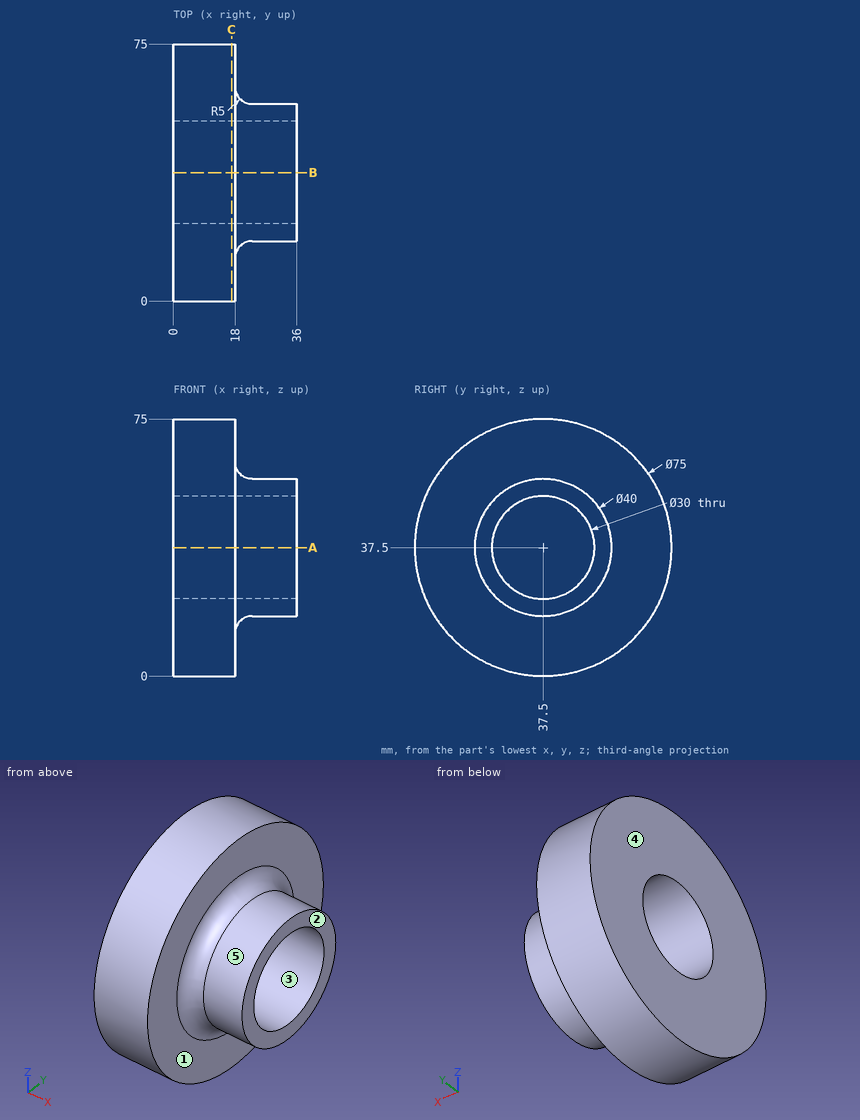
Study the drawing (mm; zero at the part's minimum x, y, z) and answer. A direction names the side the tool comes from. Round coordinates to 2 decimals unless told otherwise and drop trailing zeros. Write each loop counter-clockwise with the first axis right and the second up, starting at its lowest first coordinate (ties: lowest second). Pieces come first, ordered by that corner, then holes. Notation, with made-up numbers: (39.5, 68.25) - (93.5, 68.25) arc R19 cw to (93.5, 104.25) - close; hole circle Ø3 at (33, 10). An arc over 180 degrees is marked (long way). Return JSON: item names as keys, results as strings. Group by question number.
Q1. The part is cut by section A-A on z = 37.5. Write down the section's boundary in (x, y).
Q2. The part is cut by section C-C on x = 17. Write down the section's boundary in (y, z), then the cut area to 3 significant figures.
Q3. Each of these flat-tipped pins is pushed along its axis until it touches: pin 1 Ø4 at (x, z) = (31.5, 29) entering from -Y; pin 2 Ø3 at (x, z) = (12.5, 66.5) entering from -Y; pin 3 Ø3 at (x, z) = (28.5, 36) entering from +Y. Where does it stop, or does it pass through?
Q4. Find the intervals of material crossed by L1, parallel to Y at x = 28, z = 37; L2, parallel to Y at x = 21, z = 37; L3, parallel to X at y = 68, z = 20.5, in increasing order.
Q5. The mould has two halves that part along Y. Classify the marked faces 3, 4 and 5: released by +Y, released by -Y, zero draft, split by the parting line, or undercut.
Q6. For the marked faces 1 and 2, determine the directions among +Z, -Z, +X, -X, +Y, -Y from which every point of the face is accessible in a straight line to the end or side of a thin tool.
Solved:
{
 "1": {"outline": "(0, 0) - (18, 0) - (18, 12.5) arc R5 cw to (23, 17.5) - (36, 17.5) - (36, 22.5) - (0, 22.5) - close; (0, 52.5) - (36, 52.5) - (36, 57.5) - (23, 57.5) arc R5 cw to (18, 62.5) - (18, 75) - (0, 75) - close"},
 "2": {"outline": "circle Ø75 at (37.5, 37.5); hole circle Ø30 at (37.5, 37.5)", "area": "3,710 mm²"},
 "3": {"pin 1": "y = 18.59", "pin 2": "y = 12", "pin 3": "y = 57.5"},
 "4": {"L1": "17.51 to 22.51, 52.49 to 57.49", "L2": "17.09 to 22.51, 52.49 to 57.91", "L3": "0 to 18"},
 "5": {"face 3": "undercut", "face 4": "zero draft", "face 5": "split by the parting line"},
 "6": {"face 1": "+X", "face 2": "+Z, -Z, +X, +Y, -Y"}
}
